from build123d import *

# Parameters (mm, degrees)
SKETCH1_W           = 150
SKETCH1_H           = 130
BOSS_EXTRUDE1_DEPTH = 3
SKETCH3_W           = 50
SKETCH3_H           = 15
SKETCH3_H_2         = 16
BOSS_EXTRUDE2_DEPTH = 3
SKETCH2_R           = 1.6
CUT_EXTRUDE1_DEPTH  = 10


with BuildPart() as part:
    # Sketch1 → Boss-Extrude1 (new body)
    with BuildSketch(Plane.XY):
        Rectangle(SKETCH1_W, SKETCH1_H)
    extrude(amount=BOSS_EXTRUDE1_DEPTH)

    # Sketch3 → Boss-Extrude2 (add)
    with BuildSketch(Plane(origin=(0, 0, 0), x_dir=(-1, 0, 0), z_dir=(0, 0, -1))):
        with Locations((50, 72.5)):
            Rectangle(SKETCH3_W, SKETCH3_H)
        with Locations((50, -73)):
            Rectangle(SKETCH3_W, SKETCH3_H_2)
    extrude(amount=-BOSS_EXTRUDE2_DEPTH)

    # Sketch2 → Cut-Extrude1 (cut)
    with BuildSketch(Plane.XY.offset(3)):
        with Locations((-30.4, 58.5)):
            Circle(SKETCH2_R)
        with Locations((-68.4, 58.5)):
            Circle(SKETCH2_R)
        with Locations((-68.4, 48.5)):
            Circle(SKETCH2_R)
        with Locations((-30.4, 48.5)):
            Circle(SKETCH2_R)
        with Locations((-68.4, -48.5)):
            Circle(SKETCH2_R)
        with Locations((-68.4, -58.5)):
            Circle(SKETCH2_R)
        with Locations((-30.4, -58.5)):
            Circle(SKETCH2_R)
        with Locations((-30.4, -48.5)):
            Circle(SKETCH2_R)
        with Locations((71, -5)):
            Circle(SKETCH2_R)
        with Locations((71, 5)):
            Circle(SKETCH2_R)
        with Locations((61, -5)):
            Circle(SKETCH2_R)
        with Locations((61, 5)):
            Circle(SKETCH2_R)
        with Locations((-68.35, -34)):
            Circle(SKETCH2_R)
        with Locations((-14.35, -34)):
            Circle(SKETCH2_R)
        with Locations((-14.35, -62)):
            Circle(SKETCH2_R)
        with Locations((-14.35, 62)):
            Circle(SKETCH2_R)
        with Locations((-14.35, 34)):
            Circle(SKETCH2_R)
        with Locations((-68.35, 34)):
            Circle(SKETCH2_R)
        with Locations((45, 0)):
            Circle(SKETCH2_R)
        with Locations((5, 0)):
            Circle(SKETCH2_R)
    extrude(amount=-CUT_EXTRUDE1_DEPTH, mode=Mode.SUBTRACT)


solid = part.part
Can you work these out from the model? Positions are in its coordinate system, mm. Round coordinates to 2 decimals unless told otherwise and drop trailing zeros. Loops run counter-clockwise (first coordinate to the right, second up) from the corner with the lowest first, then second, coordinate; pieces in that order, holes last. Notation, with made-up numbers: (84.25, -33.75) - (102.25, -33.75) arc R5 ccw to (102.25, -29.75) - close; hole circle Ø9 at (34, 45). An arc over 180 degrees is marked (long way). Answer in a Markdown table with one row per item. Add a question column.
Q1. I want a section at B-B on x = 30. List the corners of the cut face in (y, z) for me.
Q2. I want a section at A-A on z = 1.55. Count the separate pieces of the cut face and the enclosed holes in it, and give its area (3 significant figures).
Q3. For pin 1 Ø3 at (x, y) = (-14.35, -62) entering from +Z; pin 2 Ø5 at (x, y) = (45, 0) entering from +Z; pin 3 Ø1.5 at (y, z) = (74, 1) entering from +X; pin 4 Ø1 at (x, z) = (37.5, 1) entering from -Y, each with a flat end and sliding along its axis, tell me the tip position at first contact or that it passes through.
Q4. I need wall thicknesses on L1, parallel to Y at x = 61, z = 1; L2, parallel to Y at x = 45, z = 1.5; L3, parallel to Y at x = 60, z = 2.65. Which ranges of each line are inside material? Lowest first, please.
A:
| question | item | result |
|---|---|---|
| 1 | outline | (-65, 0) - (65, 0) - (65, 3) - (-65, 3) - close |
| 2 | separate pieces | 1 |
| 2 | enclosed holes | 20 |
| 2 | area | 20,900 mm^2 |
| 3 | pin 1 | through |
| 3 | pin 2 | z = 3 |
| 3 | pin 3 | x = -25 |
| 3 | pin 4 | y = -65 |
| 4 | L1 | -65 to -6.6, -3.4 to 3.4, 6.6 to 65 |
| 4 | L2 | -65 to -1.6, 1.6 to 65 |
| 4 | L3 | -65 to -6.25, -3.75 to 3.75, 6.25 to 65 |
